Part print with two shaded views. Sizes in mm from the minimum x, y, z corner. A direction names the side the tool comes from. Round coordinates to 2 decimals unless told otherwise and drop trailing zeros. Order: outer loops, then holes, each group sorted by start corner. A loop starts at its lowest first (then second) coordinate and runs counter-clockwise, first axis right, second up. Notation, with made-up numbers: M -1.75,47.5 L 26.25,47.5 A19 cw 26.25,78.5 Z; hole C 26,20.5 d8. An arc over 180 degrees is marked long. Return JSON: item names as keys, results as strings. Group by question number.
Item 1: Slice it at C-C on y = 51. Write the cut outline in (x, z), then the cut area to 3 significant figures.
Item 2: Slice it at B-B on z = 12.7. Write the cut outline in (x, y).
Item 3: Slice it at A-A on x = 12.7. Write the cut outline in (y, z).
Item 4: Probe line 1 along Y through (x, z) = (14.25, 2); line 2 along Y through (x, z) = (14.5, 17.5); line 3 along Z through (x, y) = (9.5, 53.5). List the from-to ranges inside material, lowest first.
Item 5: Slice it at D-D on z = 18. Write the cut outline in (x, y), then the cut area to 3 significant figures.
Item 6: Which spindle directions (+Z, -Z, +X, -X, +Y, -Y) get a long thin tool onto all of the face, cutting with end or side? Do the marked faces 1 and 2. Say none if no direction does.
Item 7: Pin check, flat tips, straight feed: pin 1 Ø8 at (y, z) = (16.5, 11.5) entering from -X; pin 2 Ø0.8 at (x, z) = (12.5, 14) entering from -Y; pin 3 Ø2 at (y, z) = (45, 19) entering from +X; pin 4 Ø4 at (x, z) = (15.5, 15.5) entering from -Y. Stop position of each tip, or through.
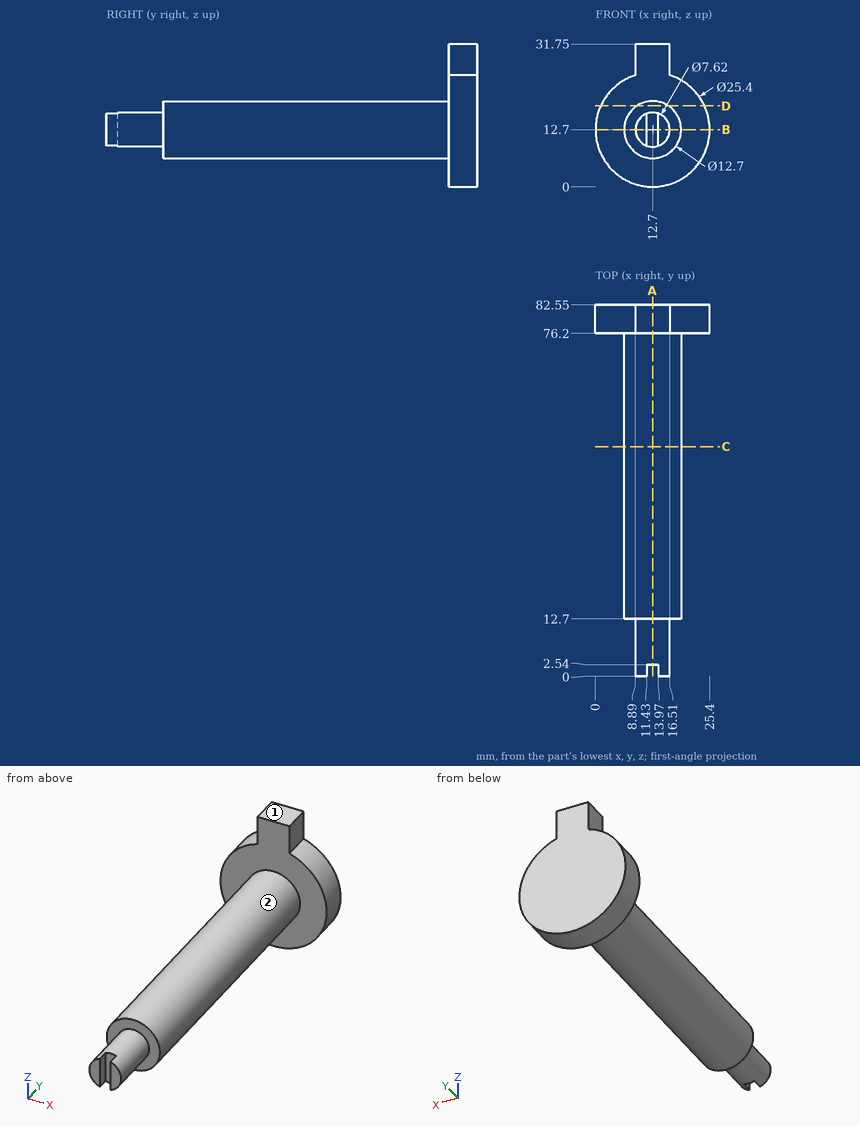
Output values:
{
 "1": {"outline": "C 12.7,12.7 d12.7", "area": "127 mm²"},
 "2": {"outline": "M 0,76.2 L 6.35,76.2 L 6.35,12.7 L 8.89,12.7 L 8.89,0 L 11.43,0 L 11.43,2.54 L 13.97,2.54 L 13.97,0 L 16.51,0 L 16.51,12.7 L 19.05,12.7 L 19.05,76.2 L 25.4,76.2 L 25.4,82.55 L 0,82.55 Z"},
 "3": {"outline": "M 2.54,8.89 L 12.7,8.89 L 12.7,6.35 L 76.2,6.35 L 76.2,0 L 82.55,0 L 82.55,31.75 L 76.2,31.75 L 76.2,19.05 L 12.7,19.05 L 12.7,16.51 L 2.54,16.51 Z"},
 "4": {"line 1": "76.2 to 82.55", "line 2": "12.7 to 82.55", "line 3": "7.22 to 18.18"},
 "5": {"outline": "M 1.16,76.2 L 9.2,76.2 L 9.2,12.7 L 16.2,12.7 L 16.2,76.2 L 24.24,76.2 L 24.24,82.55 L 1.16,82.55 Z", "area": "591 mm²"},
 "6": {"face 1": "+Z, +X, -X, +Y, -Y", "face 2": "-Y"},
 "7": {"pin 1": "x = 6.35", "pin 2": "y = 2.54", "pin 3": "x = 16.2", "pin 4": "y = 0"}
}
